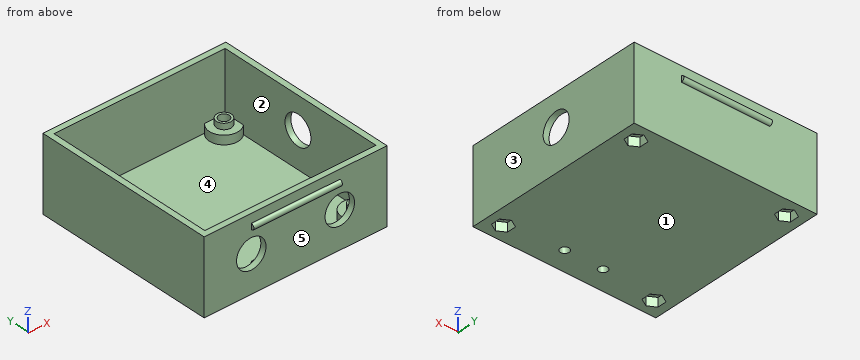
```python
from build123d import *

# Parameters (mm, degrees)
SKETCH_W        = 62
SKETCH_H        = 62
PAD_DEPTH       = 25
SKETCH001_W     = 58
SKETCH001_H     = 58
POCKET_DEPTH    = 23
SKETCH002_R     = 4.9497474683
PAD001_DEPTH    = 3
SKETCH003_R     = 2.5
PAD002_DEPTH    = 2
SKETCH004_R     = 1.75
POCKET001_DEPTH = 7.001
POCKET002_DEPTH = 3
SKETCH006_R     = 1.5
POCKET003_DEPTH = 2.001
SKETCH007_R     = 5
POCKET004_DEPTH = 2
SKETCH008_R     = 5
POCKET005_DEPTH = 2
SKETCH009_R     = 1
PAD003_DEPTH    = 15


with BuildPart() as part:
    # Sketch → Pad (new body)
    with BuildSketch(Plane.XY):
        Rectangle(SKETCH_W, SKETCH_H)
    extrude(amount=PAD_DEPTH)

    # Sketch001 (on Face6 of Pad) → Pocket (cut)
    with BuildSketch(Plane.XY.offset(25)):
        Rectangle(SKETCH001_W, SKETCH001_H)
    extrude(amount=-POCKET_DEPTH, mode=Mode.SUBTRACT)

    # Sketch002 (on Face11 of Pocket) → Pad001 (join)
    with BuildSketch(Plane.XY.offset(2)):
        with Locations((-25.5, 25.5)):
            Circle(SKETCH002_R)
        with Locations((25.5, 25.5)):
            Circle(SKETCH002_R)
        with Locations((25.5, -25.5)):
            Circle(SKETCH002_R)
        with Locations((-25.5, -25.5)):
            Circle(SKETCH002_R)
    extrude(amount=PAD001_DEPTH)

    # Sketch003 (on Face15 of Pad001) → Pad002 (join)
    with BuildSketch(Plane.XY.offset(5)):
        with Locations((-25.5, 25.5)):
            Circle(SKETCH003_R)
        with Locations((25.5, 25.5)):
            Circle(SKETCH003_R)
        with Locations((25.5, -25.5)):
            Circle(SKETCH003_R)
        with Locations((-25.5, -25.5)):
            Circle(SKETCH003_R)
    extrude(amount=PAD002_DEPTH)

    # Sketch004 (on Face27 of Pad002) → Pocket001 (cut, through all)
    with BuildSketch(Plane.XY.offset(7)):
        with Locations((-25.5, 25.5)):
            Circle(SKETCH004_R)
        with Locations((25.5, 25.5)):
            Circle(SKETCH004_R)
        with Locations((25.5, -25.5)):
            Circle(SKETCH004_R)
        with Locations((-25.5, -25.5)):
            Circle(SKETCH004_R)
    extrude(amount=-POCKET001_DEPTH, mode=Mode.SUBTRACT)

    # Sketch005 (on Face4 of Pocket001) → Pocket002 (cut)
    with BuildSketch(Plane(origin=(0, 0, 0), x_dir=(1, 0, 0), z_dir=(0, 0, -1))):
        Polygon((-22.8, 23.9411542732), (-22.8, 27.0588457268), (-25.5, 28.6176914536), (-28.2, 27.0588457268), (-28.2, 23.9411542732), (-25.5, 22.3823085464), align=None)
        Polygon((22.8, 23.9411542732), (25.5, 22.3823085464), (28.2, 23.9411542732), (28.2, 27.0588457268), (25.5, 28.6176914536), (22.8, 27.0588457268), align=None)
        Polygon((-22.8, -27.0588457268), (-22.8, -23.9411542732), (-25.5, -22.3823085464), (-28.2, -23.9411542732), (-28.2, -27.0588457268), (-25.5, -28.6176914536), align=None)
        Polygon((25.5, -28.6176914536), (28.2, -27.0588457268), (28.2, -23.9411542732), (25.5, -22.3823085464), (22.8, -23.9411542732), (22.8, -27.0588457268), align=None)
    extrude(amount=-POCKET002_DEPTH, mode=Mode.SUBTRACT)

    # Sketch006 (on Face41 of Pocket002) → Pocket003 (cut, through all)
    with BuildSketch(Plane.XY.offset(2)):
        with Locations((-6.5, -23.5)):
            Circle(SKETCH006_R)
        with Locations((6.5, -23.5)):
            Circle(SKETCH006_R)
    extrude(amount=-POCKET003_DEPTH, mode=Mode.SUBTRACT)

    # Sketch007 (on Face6 of Pocket003) → Pocket004 (cut)
    with BuildSketch(Plane.XZ.offset(31)):
        with Locations((-15, 12.5)):
            Circle(SKETCH007_R)
        with Locations((15, 12.5)):
            Circle(SKETCH007_R)
    extrude(amount=-POCKET004_DEPTH, mode=Mode.SUBTRACT)

    # Sketch008 (on Face3 of Pocket004) → Pocket005 (cut)
    with BuildSketch(Plane.YZ.offset(31)):
        with Locations((1, 14.2)):
            Circle(SKETCH008_R)
    extrude(amount=-POCKET005_DEPTH, mode=Mode.SUBTRACT)

    # Sketch009 (on DatumPlane) → Pad003 (join, symmetric)
    with BuildSketch(Plane(origin=(0, -31, 25), x_dir=(0, 1, 0), z_dir=(1, 0, 0))):
        with Locations((0, -4.1)):
            Circle(SKETCH009_R)
        with Locations((62, -4.1)):
            Circle(SKETCH009_R)
    extrude(amount=PAD003_DEPTH, both=True)


solid = part.part
```
Geometry check sheet. Reference: the model listing, model coordinates, mm. Face numbers are marked on the shaded views. A direction names the side the tool comes from. Give positions to 0.01 mm unless a question says otherwise; leave off trailing zeros. Order: outer loops, then holes, each group sorted by start corner. A loop starts at its lowest first (then second) coordinate and runs counter-clockwise, first axis right, second up.
1. Section check B-B, the plane z = 20.9. Enter the section's corners in (x, y), and give its area (3 significant figures).
2. Section check C-C, the plane z = 14.2. Enter the section's corners in (x, y).
3. Access from +Z, -Z, +X, -X, +Y, -Y to the whole of each face (thin tool, end or side, straight path). Record for the marked faces 1 and 2.
4. Section check A-A, the plane x = 6.5. Enter the section's corners in (y, z), and give its area (3 significant figures).
5. Release check for a two-part mould opening along Y. For the marked faces 3, 4 and 5 record: pulls with the +Y half, pulls with the -Y half, needs draft (parallel to the pull), parting line crosses it, or undercut.
6. Section check D-D, the plane y = 8.5. Enter the section's corners in (x, z), and give its area (3 significant figures).
7. Gauge pin test, flat ends, axial feed: pin 1 Ø0.5 at (y, z) = (31.5, 21) entering from +X; pin 2 Ø3.5 at (x, y) = (-6.5, -23.5) entering from -Z; pin 3 Ø4.5 at (x, y) = (-25.5, -25.5) entering from +Z; pin 4 Ø6 at (x, y) = (-16.5, -2.5) entering from +Z. Record the tip position at first contact, or that the pin passes through.
8. Thickness scan on L1, parallel to Y at x = -25.5, z = 5.9; L2, parallel to Y at x = 23.5, z = 18.75; L3, parallel to Y at x = 23, z = 2.25. Record the ranges inside material, lowest first.
Values follow:
1. outline: (-31, -31) - (-15, -31) - (-15, -32) - (15, -32) - (15, -31) - (31, -31) - (31, 31) - (15, 31) - (15, 32) - (-15, 32) - (-15, 31) - (-31, 31) - close; hole (-29, -29) - (29, -29) - (29, 29) - (-29, 29) - close
1. area: 540 mm2
2. outline: (-31, -31) - (-19.7, -31) - (-19.7, -29) - (-29, -29) - (-29, 29) - (29, 29) - (29, 6) - (31, 6) - (31, 31) - (-31, 31) - close; (-10.3, -31) - (10.3, -31) - (10.3, -29) - (-10.3, -29) - close; (19.7, -31) - (31, -31) - (31, -4) - (29, -4) - (29, -29) - (19.7, -29) - close
3. face 1: -Z, +X, -X, +Y, -Y
3. face 2: +Z
4. outline: (-31, 0) - (-25, 0) - (-25, 2) - (-29, 2) - (-29, 25) - (-31, 25) - (-31, 21.9) arc R1 ccw to (-31, 19.9) - close; (-22, 0) - (31, 0) - (31, 19.9) arc R1 ccw to (31, 21.9) - (31, 25) - (29, 25) - (29, 2) - (-22, 2) - close
4. area: 213 mm2
5. face 3: needs draft
5. face 4: undercut
5. face 5: pulls with the -Y half
6. outline: (-31, 0) - (31, 0) - (31, 25) - (29, 25) - (29, 2) - (-29, 2) - (-29, 25) - (-31, 25) - close
6. area: 216 mm2
7. pin 1: stops at x = 15
7. pin 2: stops at z = 0
7. pin 3: stops at z = 7
7. pin 4: stops at z = 2
8. L1: y = -31 to -29, -28 to -27.25, -23.75 to -23, 23 to 23.75, 27.25 to 28, 29 to 31
8. L2: y = -31 to -29, 29 to 31
8. L3: y = -31 to -27.17, -23.83 to -21.23, 21.23 to 23.83, 27.17 to 31
